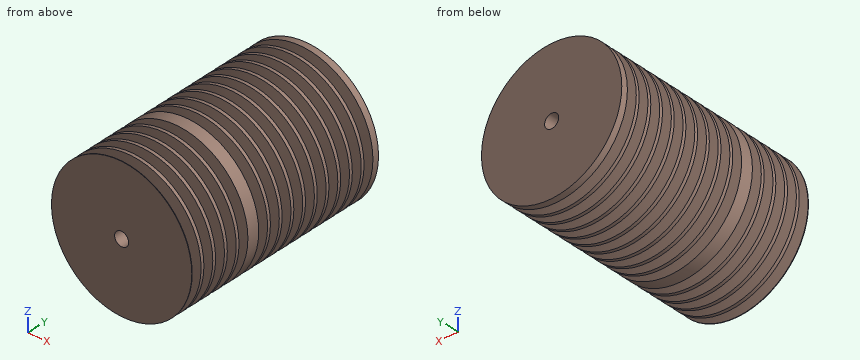
```python
from build123d import *

# Parameters (mm, degrees)
F0_R        = 63.5
F0_R_2      = 6.35
F1_DEPTH    = 127
F1_FACE_R   = 63.5
F1_FACE_R_2 = 6.35
F4_DEPTH    = 63.5


with BuildPart() as f1:
    # F0 (on Front) → F1 (new body)
    with BuildSketch(Plane.XZ):
        Circle(F0_R)
        Circle(F0_R_2, mode=Mode.SUBTRACT)
    extrude(amount=F1_DEPTH)

    # F2 (on Right) → F3 (revolve, cut)
    with BuildSketch(Plane.YZ):
        Polygon((-10.730011, 43.902457), (-5.359275, 64.943254), (-11.938, 64.943254), (-15.07775, 64.943254), align=None)
        Polygon((-22.668011, 43.902457), (-17.297275, 64.943254), (-23.876, 64.943254), (-27.01575, 64.943254), align=None)
        Polygon((-34.606011, 43.902457), (-29.235275, 64.943254), (-35.814, 64.943254), (-38.95375, 64.943254), align=None)
        Polygon((-46.544011, 43.902457), (-41.173275, 64.943254), (-47.752, 64.943254), (-50.89175, 64.943254), align=None)
        Polygon((-58.482011, 43.902457), (-53.111275, 64.943254), (-59.69, 64.943254), (-62.82975, 64.943254), align=None)
        Polygon((-70.420011, 43.902457), (-65.049275, 64.943254), (-71.628, 64.943254), (-74.76775, 64.943254), align=None)
        Polygon((-82.358011, 43.902457), (-76.987275, 64.943254), (-83.566, 64.943254), (-86.70575, 64.943254), align=None)
        Polygon((-94.296011, 43.902457), (-88.925275, 64.943254), (-95.504, 64.943254), (-98.64375, 64.943254), align=None)
        Polygon((-106.234011, 43.902457), (-100.863275, 64.943254), (-107.442, 64.943254), (-110.58175, 64.943254), align=None)
        Polygon((-118.172011, 43.902457), (-112.801275, 64.943254), (-122.51975, 64.943254), align=None)
        Polygon((-137.317755, 43.902457), (-132.970016, 64.943254), (-139.682883, 64.943254), (-142.688491, 64.943254), align=None)
        Polygon((-149.255755, 43.902457), (-144.908016, 64.943254), (-151.620883, 64.943254), (-154.626491, 64.943254), align=None)
        Polygon((-161.193755, 43.902457), (-156.846016, 64.943254), (-163.558883, 64.943254), (-166.564491, 64.943254), align=None)
        Polygon((-173.131755, 43.902457), (-168.784016, 64.943254), (-175.496883, 64.943254), (-178.502491, 64.943254), align=None)
        Polygon((-185.069755, 43.902457), (-180.722016, 64.943254), (-187.434883, 64.943254), (-190.440491, 64.943254), align=None)
        Polygon((-197.007755, 43.902457), (-192.660016, 64.943254), (-199.372883, 64.943254), (-202.378491, 64.943254), align=None)
    revolve(axis=Axis((0, -127, 0), (0, -1, 0)), mode=Mode.SUBTRACT)

    # F1_face (on face) → F4 (join)
    with BuildSketch(Plane.XZ.offset(127)):
        Circle(F1_FACE_R)
        Circle(F1_FACE_R_2, mode=Mode.SUBTRACT)
    extrude(amount=F4_DEPTH)

    # F2 (on Right) → F5 (revolve, cut)
    with BuildSketch(Plane.YZ):
        Polygon((-137.317755, 43.902457), (-132.970016, 64.943254), (-139.682883, 64.943254), (-142.688491, 64.943254), align=None)
        Polygon((-10.730011, 43.902457), (-5.359275, 64.943254), (-11.938, 64.943254), (-15.07775, 64.943254), align=None)
        Polygon((-220.883755, 43.902457), (-216.536016, 64.943254), (-223.248883, 64.943254), (-226.254491, 64.943254), align=None)
        Polygon((-208.945755, 43.902457), (-204.598016, 64.943254), (-211.310883, 64.943254), (-214.316491, 64.943254), align=None)
        Polygon((-197.007755, 43.902457), (-192.660016, 64.943254), (-199.372883, 64.943254), (-202.378491, 64.943254), align=None)
        Polygon((-185.069755, 43.902457), (-180.722016, 64.943254), (-187.434883, 64.943254), (-190.440491, 64.943254), align=None)
        Polygon((-173.131755, 43.902457), (-168.784016, 64.943254), (-175.496883, 64.943254), (-178.502491, 64.943254), align=None)
        Polygon((-161.193755, 43.902457), (-156.846016, 64.943254), (-163.558883, 64.943254), (-166.564491, 64.943254), align=None)
        Polygon((-149.255755, 43.902457), (-144.908016, 64.943254), (-151.620883, 64.943254), (-154.626491, 64.943254), align=None)
        Polygon((-118.172011, 43.902457), (-112.801275, 64.943254), (-122.51975, 64.943254), align=None)
        Polygon((-106.234011, 43.902457), (-100.863275, 64.943254), (-107.442, 64.943254), (-110.58175, 64.943254), align=None)
        Polygon((-94.296011, 43.902457), (-88.925275, 64.943254), (-95.504, 64.943254), (-98.64375, 64.943254), align=None)
        Polygon((-82.358011, 43.902457), (-76.987275, 64.943254), (-83.566, 64.943254), (-86.70575, 64.943254), align=None)
        Polygon((-70.420011, 43.902457), (-65.049275, 64.943254), (-71.628, 64.943254), (-74.76775, 64.943254), align=None)
        Polygon((-58.482011, 43.902457), (-53.111275, 64.943254), (-59.69, 64.943254), (-62.82975, 64.943254), align=None)
        Polygon((-46.544011, 43.902457), (-41.173275, 64.943254), (-47.752, 64.943254), (-50.89175, 64.943254), align=None)
        Polygon((-34.606011, 43.902457), (-29.235275, 64.943254), (-35.814, 64.943254), (-38.95375, 64.943254), align=None)
        Polygon((-22.668011, 43.902457), (-17.297275, 64.943254), (-23.876, 64.943254), (-27.01575, 64.943254), align=None)
    revolve(axis=Axis((0, -62.531525, 0), (0, 1, 0)), mode=Mode.SUBTRACT)


solid = f1.part
```
Geometry: final body of the model. Coordinates: model frame, mm. Give positions to 0.01 mm unless a question says otherwise; leave off trailing zeros.
1. Pin query (flat end, axial travel): P1, Ø5, axis at y = -164, z = 21, coming from the +X side; P2, Ø10, axis at x = -26, z = -6, coming from the +Y side; P3, Ø8, axis at y = -26.5, z = 11.5, coming from the -X side; P4, Ø12, axis at y = -150.5, z = -37, coming from the +X side. Return the tip coordinate at first contact, or that it passes through.
2. Section query A-A, the plane x = -49.5. Count the separate pieces of the cut face and the enclosed holes in it, then the cut area to 3 significant figures.
3. Line query: probe 1 along Z at (x, y) = (0, -145); probe 2 along Z at (x, y) = (19, -111.5); probe 3 along Z at (x, y) = (44, -100). Output: solid intervals per line, ascending.
Computed:
1. P1: stops at x = 60.33
1. P2: stops at y = 0
1. P3: stops at x = -63.05
1. P4: stops at x = 54.66
2. separate pieces: 16
2. enclosed holes: 0
2. area: 9,370 mm2
3. probe 1: z = -63.5 to -6.35, 6.35 to 63.5
3. probe 2: z = -60.59 to 60.59
3. probe 3: z = -45.78 to 45.78
